Print and shaded views of the part. All mm, measured from the part's lowest x, y and z. A direction names the side the tool comes from. Round coordinates to 2 decimals unless told otherwise and drop trailing zeros. Order: outer loops, then holes, each group sorted by start corner. A loop starts at its lowest first (then second) coordinate and runs counter-clockwise, first axis right, second up. Notation, with made-up numbers: (-9.75, 84) -> (47.25, 84) arc R18 ccw to (47.25, 114) -> close; hole circle Ø7 at (1.5, -29.5). An arc over 180 degrees is marked (long way). Answer as CSV lines item,"result".
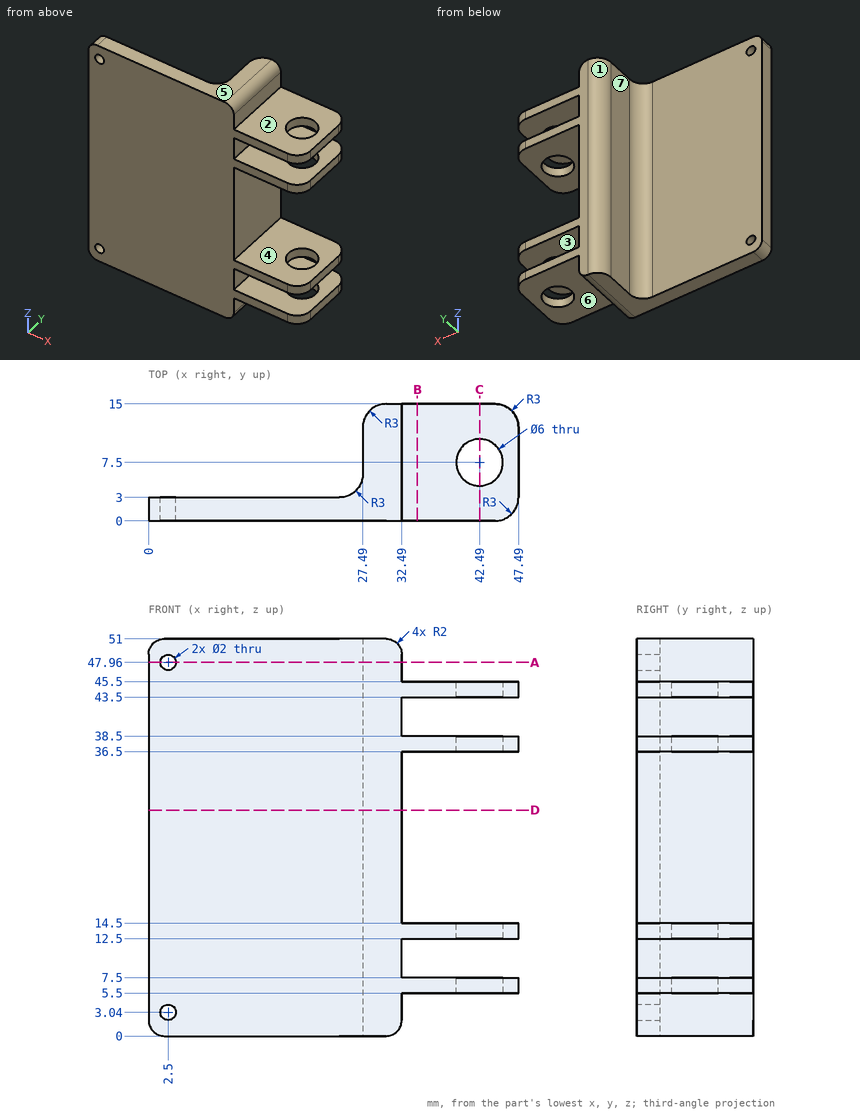
Q1. Saw through at B-B (x = 34.5). Write the cut outline in (y, z).
Checks:
outline,"(0, 5.5) -> (15, 5.5) -> (15, 7.5) -> (0, 7.5) -> close; (0, 12.5) -> (15, 12.5) -> (15, 14.5) -> (0, 14.5) -> close; (0, 36.5) -> (15, 36.5) -> (15, 38.5) -> (0, 38.5) -> close; (0, 43.5) -> (15, 43.5) -> (15, 45.5) -> (0, 45.5) -> close"
Q2. Saw through at A-A (z = 47.96). Write the cut outline in (x, y).
Checks:
outline,"(0, 0) -> (1.5, 0) -> (1.5, 3) -> (0, 3) -> close; (3.5, 0) -> (32.49, 0) -> (32.49, 15) -> (30.49, 15) arc R3 ccw to (27.49, 12) -> (27.49, 6) arc R3 cw to (24.49, 3) -> (3.5, 3) -> close"
Q3. Tool access for the marked faces 4, 5, 6 and 7: list every direction of +Z, -Z, +X, -X, +Y, -Y with a clear straight run to the whole face (end or side of a thin tool).
Checks:
face 4,"+X, +Y, -Y"
face 5,"+Z, +X, -X, +Y, -Y"
face 6,"-Z, +X, +Y, -Y"
face 7,"+Z, -Z, -X, +Y"
Q4. Saw through at D-D (z = 29). Write the cut outline in (x, y), plus the area to 3 significant figures.
Checks:
outline,"(0, 0) -> (32.49, 0) -> (32.49, 15) -> (30.49, 15) arc R3 ccw to (27.49, 12) -> (27.49, 6) arc R3 cw to (24.49, 3) -> (0, 3) -> close"
area,"157 mm²"
Q5. Saw through at C-C (x = 42.49). State how many separate pieces and enclosed holes the cut face has, plus the area to 3 significant figures.
Checks:
separate pieces,"8"
enclosed holes,"0"
area,"72.0 mm²"
Q6. Wall check: L1, parallel to Z at x = 35, y = 5; L2, parallel to Y at x = 42.49, z = 14; L3, parallel to X at y = 2.2, z = 47.96. Give the ranges that are in metal, low to high. Write a range as [from, to].
Checks:
L1,"[5.5, 7.5], [12.5, 14.5], [36.5, 38.5], [43.5, 45.5]"
L2,"[0, 4.5], [10.5, 15]"
L3,"[0, 1.5], [3.5, 32.49]"
Q7. Mould opens along Z. For the marked faces 1, 2 and 3 say: +Z half, -Z half, draft (parallel to the pull), parting line (faces both ways), or undercut.
Checks:
face 1,"draft"
face 2,"+Z half"
face 3,"undercut"
Q8. Flat gauge pins, fed straight in: pin 1 (2.5 mm diameter, centred on x = 2.5, z = 47.96, fed in from +Y); pin 2 (1.8 mm diameter, centred on y = 9.5, z = 4, fed in from +X); pin 3 (4.5 mm diameter, centred on x = 36.5, y = 5, fed in from +Z). Where does each tip first touch, or does it go through?
Checks:
pin 1,"y = 3"
pin 2,"x = 32.49"
pin 3,"z = 45.5"
